Design review of the part built by this model. Coordinates are the model's own, in mm. Coordinates: 2 decimals unless noted, no trailing zeros. Write each loop counter-clockwise with the first axis right and the second up, starting at its lowest first coordinate (ties: lowest second). Pieces come first, ordered by that corner, then holes. Notation, with made-up numbers: (89.25, 19) - (133.25, 19) arc R6 ccw to (133.25, 26) - close; hole circle Ø5 at (76, 30.25). An arc over 180 degrees is marked (long way). One line per item, written item: value.
from build123d import *

# Parameters (mm, degrees)
CUT_EXTRUDE1_DEPTH      = 90.044932478
CUT_EXTRUDE1_DEPTH_BACK = 90.044932478
SKETCH3_R               = 1


with BuildPart() as part:
    # Sketch1 → Revolve1 (revolve)
    with BuildSketch(Plane.XY, mode=Mode.PRIVATE) as revolve1_sk:
        Polygon((0, 1.5), (-6, 1.5), (-6, 0), (89, 0), (89, 2), (0, 2), align=None)
    revolve(revolve1_sk.sketch.rotate(Axis((-6, 0, 0), (1, 0, 0)), 180), axis=Axis((-6, 0, 0), (1, 0, 0)))

    # Sketch3 → Cut-Extrude1 (cut, two sides: drawn at the far end of the back side and taken through both)
    with BuildSketch(Plane(origin=(0, 0, 0), x_dir=(1, 0, 0), z_dir=(0, 1, 0)).offset(-CUT_EXTRUDE1_DEPTH_BACK)):
        with Locations(Location((3, 0, 0), (0, 0, 270))):
            Circle(SKETCH3_R)
        with Locations(Location((78, 0, 0), (0, 0, 270))):
            Circle(SKETCH3_R)
    extrude(amount=CUT_EXTRUDE1_DEPTH + CUT_EXTRUDE1_DEPTH_BACK, mode=Mode.SUBTRACT)


solid = part.part
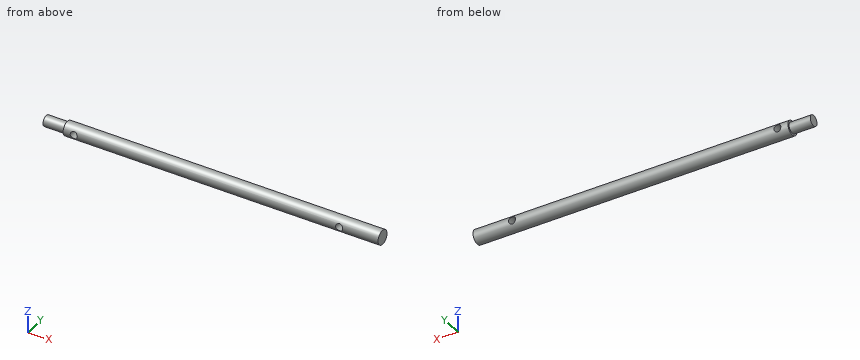
1. Consider section A-A, the plane y = 0. Write out the cut boundary in (x, z).
Answer block:
outline: (-6, -1.5) - (0, -1.5) - (0, -2) - (89, -2) - (89, 2) - (0, 2) - (0, 1.5) - (-6, 1.5) - close; hole circle Ø2 at (3, 0); hole circle Ø2 at (78, 0)
2. Insertion check: pin 1 Ø1.5 at (x, z) = (6.5, -1) entering from -Y; pin 2 Ø1.6 at (x, z) = (3, 0) entering from -Y; pin 3 Ø1 at (x, y) = (63, 1) entering from +Z. Each pin has a flat end and moves straight along its axis. Give the tip position at first contact, or say it passes through.
Answer block:
pin 1: stops at y = -1.98
pin 2: passes through
pin 3: stops at z = 1.94
3. Consider section B-B, the plane x = 3. Write out the cut boundary in (y, z), then the cut area to 3 significant figures.
Answer block:
outline: (-1.73, -1) arc R2 ccw to (1.73, -1) - close; (-1.73, 1) - (1.73, 1) arc R2 ccw to start
area: 4.91 mm^2
4. Wall thickness on line 1 along X through (y, z) = (-0.25, 0); line 2 along Z through (x, y) = (3, -0.15); line 3 along X through (y, z) = (-0.6, 0.5): over which ranges is each line inside the solid? List them lowest first.
Answer block:
line 1: x = -6 to 2, 4 to 77, 79 to 89
line 2: z = -1.99 to -1, 1 to 1.99
line 3: x = -6 to 2.13, 3.87 to 77.13, 78.87 to 89
